Work out the finished part from the listing and answer in its coordinate system (mm). A direction names the side the tool comes from. Round coordinates to 2 decimals unless told otherwise and drop trailing zeros. Loops run counter-clockwise (first coordinate to the right, second up) from the corner with the lowest first, then second, coordinate; pieces in that order, holes last. Notation, with made-up numbers: (-24, 7) - (-16, 7) arc R26 cw to (-16, 26) - close; hole circle Ø3 at (66, 60). An arc over 180 degrees is marked (long way). Answer as CSV lines item,"result". Start each with the question number.
Q1. The mould has two halves that part along X. Classify faces 1 (the face through (8.715, 25.709, 0.811)), 2 (the face through (0, 14.2, 1.6)), 3 (the face through (-10.227, 24, 1)): +X half, -X half, draft (parallel to the pull), parting line (faces both ways), or undercut.
Q2. Straight lines are drawn through the part: L1, parallel to X at y = 19, z = 0.75; L2, parallel to X at y = 9.75, z = 0.1; L3, parallel to Y at x = -9.5, z = 1.05. For each, find the intervals that lie inside material, in ascending order. Write a range as [from, to].
Q3. Section C-C on y = 15.25 is taken. Write down the section's boundary in (x, z), then the cut area to 3 significant figures.
Q4. For faces 4 (the face through (7.47, 27.66, 0.79)), 5 (the face through (-8, 17, 1)), 6 (the face through (5.97, 7.6, 0.79)), 7 (the face through (1.723, 2.47, 0.811)), determine the directions among +Z, -Z, +X, -X, +Y, -Y from which every point of the face is accessible in a straight line to the end or side of a thin tool.
Q5. Section A-A on y = 19 is taken. Write down the section's boundary in (x, z), then the cut area to 3 significant figures.
Q6. Each of these flat-tipped pins is pushed along its axis until it touches: pin 1 Ø0.5 at (x, z) = (0, 1) entering from +Y; pin 2 Ø0.5 at (x, z) = (6, 1) entering from +Y; pin 3 Ø1.5 at (x, y) = (1.5, 5.5) entering from -Z. Where does it stop, or does it pass through?
Q7. Section B-B on x = -0.75 is taken. Write down the section's boundary in (y, z), then the cut area to 3 significant figures.
```python
from build123d import *

# Parameters (mm, degrees)
BOSS_EXTRUDE1_DEPTH = 1.6
FILLET7_R           = 0.5
FILLET8_R           = 2.5
FILLET9_R           = 2.5
MIRROR1_DEPTH       = 1.6
FILLET10_R          = 1


# Read off the part's stored shape, not the designer's step: Mirror1
with BuildPart() as part:
    # Sketch1 → Boss-Extrude1 (new body)
    with BuildSketch(Plane.XY):
        Polygon((5, 16), (0, 16), (0, 14), (5.901749013, 14), (2.094432467, 2), (0, 2), (0, 0), (3.558130696, 0), (8, 14), (8, 20.3), (10.226542067, 20.3), (10.226542067, 28.3), (6.6499, 28.3), (6.6499, 26.01), (9, 26.01), (9, 24), (6.6499, 24), (6.6499, 21.5), (5, 21.5), align=None)
    extrude(amount=BOSS_EXTRUDE1_DEPTH)

    # Fillet7
    fillet7_edges = [part.edges().sort_by_distance(p)[0] for p in [
        (5, 16, 0.8),
        (5, 21.5, 0.8),
        (6.6499, 21.5, 0.8),
        (10.226542067, 28.3, 0.8),
        (10.226542067, 20.3, 0.8),
        (8, 20.3, 0.8),
    ]]
    fillet(fillet7_edges, radius=FILLET7_R)

    # Fillet8
    # the kernel refuses this fillet: 2.5 mm, written as the material it takes off along each edge
    with BuildSketch(Plane(origin=(6.6499, 28.3, -6.227910966), x_dir=(0, -1, 0), z_dir=(0, 0, 1))) as fillet8_piece_1:
        with BuildLine():
            CenterArc((2.5, 2.491164386), FILLET8_R, 180, 85.181476567)
            Line((0, 2.491164386), (-0.05, 2.491164386))
            Line((-0.05, 2.491164386), (-0.05, 0))
            Line((-0.05, 0), (0, -0.05))
            ThreePointArc((0, -0.05), (1.145, -0.05), (2.2858, -0.049823288))
            Line((2.2858, -0.049823288), (2.29, 0))
        make_face()
    extrude(amount=14.055821932, mode=Mode.SUBTRACT)

    # Fillet9
    fillet9_edges = [part.edges().sort_by_distance(p)[0] for p in [
        (8, 14, 0.8),
        (3.558130696, 0, 0.8),
        (2.094432467, 2, 0.8),
        (5.901749013, 14, 0.8),
    ]]
    fillet(fillet9_edges, radius=FILLET9_R)

    # Mirror1 outline → Mirror1 (add)
    with BuildSketch(Plane.XY):
        with BuildLine():
            Line((0, 16), (-4.5, 16))
            ThreePointArc((-4.5, 16), (-4.853553391, 16.146446609), (-5, 16.5))
            Line((-5, 16.5), (-5, 21))
            ThreePointArc((-5, 21), (-5.146446609, 21.353553391), (-5.5, 21.5))
            Line((-5.5, 21.5), (-6.1499, 21.5))
            ThreePointArc((-6.1499, 21.5), (-6.503453391, 21.646446609), (-6.6499, 22))
            Line((-6.6499, 22), (-6.6499, 24))
            Line((-6.6499, 24), (-9, 24))
            Line((-9, 24), (-9, 26.01))
            Line((-9, 26.01), (-6.6499, 26.01))
            ThreePointArc((-6.6499, 26.01), (-7.449171955, 27.640516232), (-9.141064386, 28.3))
            Line((-9.141064386, 28.3), (-9.726542067, 28.3))
            ThreePointArc((-9.726542067, 28.3), (-10.080095458, 28.153553391), (-10.226542067, 27.8))
            Line((-10.226542067, 27.8), (-10.226542067, 20.8))
            ThreePointArc((-10.226542067, 20.8), (-10.080095458, 20.44644661), (-9.726542067, 20.3))
            Line((-9.726542067, 20.3), (-8.5, 20.3))
            ThreePointArc((-8.5, 20.3), (-8.146446609, 20.153553391), (-8, 19.8))
            Line((-8, 19.8), (-8, 14.38708754))
            ThreePointArc((-8, 14.38708754), (-7.970560929, 14.004558199), (-7.882937042, 13.631037905))
            Line((-7.882937042, 13.631037905), (-4.111444952, 1.743950364))
            ThreePointArc((-4.111444952, 1.743950364), (-3.204969205, 0.482560523), (-1.72850791, 0))
            Line((-1.72850791, 0), (0, 0))
            Line((0, 0), (0, 2))
            Line((0, 2), (-0.264809681, 2))
            ThreePointArc((-0.264809681, 2), (-1.741270976, 2.482560523), (-2.647746723, 3.743950364))
            Line((-2.647746723, 3.743950364), (-4.868681376, 10.743950364))
            ThreePointArc((-4.868681376, 10.743950364), (-4.503183811, 12.976461295), (-2.485744333, 14))
            Line((-2.485744333, 14), (0, 14))
            Line((0, 14), (0, 16))
        make_face()
    extrude(amount=MIRROR1_DEPTH)

    # Fillet10
    fillet10_edges = [part.edges().sort_by_distance(p)[0] for p in [
        (-9, 24, 0.8),
        (-9, 26.01, 0.8),
        (9, 24, 0.8),
        (9, 26.01, 0.8),
    ]]
    fillet(fillet10_edges, radius=FILLET10_R)


solid = part.part
```
Findings:
1,face 1,"undercut"
1,face 2,"draft"
1,face 3,"-X half"
2,L1,"x = [-8, -5], [5, 8]"
2,L2,"x = [-6.65, -4.55], [4.55, 6.65]"
2,L3,"y = [20.3, 28.3]"
3,outline,"(-8, 0) - (8, 0) - (8, 1.6) - (-8, 1.6) - close"
3,area,"25.6 mm^2"
4,face 4,"+Z, -Z, +Y"
4,face 5,"+Z, -Z, -X, -Y"
4,face 6,"+Z, -Z, +X, -Y"
4,face 7,"+Z, -Z"
5,outline,"(-8, 0) - (-5, 0) - (-5, 1.6) - (-8, 1.6) - close; (5, 0) - (8, 0) - (8, 1.6) - (5, 1.6) - close"
5,area,"9.60 mm^2"
6,pin 1,"stops at y = 16"
6,pin 2,"stops at y = 21.51"
6,pin 3,"passes through"
7,outline,"(0, 0) - (2.05, 0) - (2.05, 1.6) - (0, 1.6) - close; (14, 0) - (16, 0) - (16, 1.6) - (14, 1.6) - close"
7,area,"6.48 mm^2"
